Here's how the part is built. I have some questions about the finished solid (model axes, mm). A direction names the side the tool comes from. Give positions to 0.01 mm unless a question says otherwise; leave off trailing zeros. Write each loop counter-clockwise with the first axis right and the second up, starting at its lowest first coordinate (ties: lowest second). Pieces come first, ordered by that corner, then holes. Notation, with made-up numbers: (65, 41.5) -> (81, 41.5) arc R26 cw to (81, 80.5) -> close; hole circle Ø7 at (13.25, 32). An arc over 180 degrees is marked (long way). Use CSV: the item, a comma, the result in double quotes. Start each with the question number.
(1) For pin 1 Ø1 at (y, z) = (567, 48.5) entering from -X; pin 2 Ø21 at (x, y) = (339, 296) entering from +Z; pin 3 Ø21 at (x, y) = (336, 444) entering from -Z, each with a flat end and sliding along its axis, tell me the tip position at first contact or that it passes through.
(2) I need wall thicknesses on L1, parallel to X at y = 644.5, z = -14; L2, parallel to X at y = 35, z = 18.5; L3, parallel to Y at x = -117.5, z = -49.5. Which ranges of each line are inside material? Lowest first, please. Write a range as [from, to].
(3) Suppose I cut it at C-C on x = -142.5. List the corners of the cut face in (y, z) for me, plus the area to 3 significant figures.
(4) Which directions (+Z, -Z, +X, -X, +Y, -Y) give clear straight access to the entire face, cutting with the end or side of a thin tool? Please do faces 1 (the flat face through (364, 345, 28.85)), 2 (the flat face through (338, 345, 48.85)), 3 (the flat face through (338, 345, -31.15)).
(5) Suppose I cut it at B-B on z = 11. List the corners of the cut face in (x, y) for me, plus the area to 3 significant figures.
(6) Suppose I cut it at D-D on z = -52.5. List the corners of the cut face in (x, y) for me, plus the area to 3 significant figures.
(7) If we mould it in two halves opening along X, with no side actions, what happens to faces 4 (the flat face through (345, 698.9, 9)), 5 (the flat face through (-324.85, 345, 9)), 6 (the flat face through (350.95, 345, 39))? For each: pulls with the +X half, pulls with the -X half, needs draft (parallel to the pull), parting line crosses it, or undercut.
(8) Suppose I cut it at A-A on y = 478. List the corners of the cut face in (x, z) for me.
from build123d import *

# Parameters (mm, degrees)
F0_W     = 780.2
F0_H     = 122.3
F1_DEPTH = 26.1
F2_W     = 25
F2_H     = 40
F3_DEPTH = 698.9


with BuildPart() as f1:
    # F0 (on Front) → F1 (new body)
    with BuildSketch(Plane.XZ):
        Rectangle(F0_W, F0_H)
    extrude(amount=F1_DEPTH)

    # F2 (on face) → F3 (join)
    with BuildSketch(Plane(origin=(0, 0, 0), x_dir=(-1, 0, 0), z_dir=(0, 1, 0))):
        Polygon((-350.95, 48.85), (-350.95, 28.85), (-350.95, -11.15), (-350.95, -31.15), (-324.85, -31.15), (-324.85, 48.85), align=None)
        Polygon((350.95, 28.85), (350.95, 48.85), (324.85, 48.85), (324.85, -31.15), (350.95, -31.15), (350.95, -11.15), align=None)
        with Locations((363.45, 8.85)):
            Rectangle(F2_W, F2_H)
        with Locations((-363.45, 8.85)):
            Rectangle(F2_W, F2_H)
    extrude(amount=F3_DEPTH)


solid = f1.part
Geometry says:
1,pin 1,"x = -350.95"
1,pin 2,"z = 48.85"
1,pin 3,"z = -31.15"
2,L1,"[-350.95, -324.85], [324.85, 350.95]"
2,L2,"[-375.95, -324.85], [324.85, 375.95]"
2,L3,"[-26.1, 0]"
3,outline,"(-26.1, -61.15) -> (0, -61.15) -> (0, 61.15) -> (-26.1, 61.15) -> close"
3,area,"3,190 mm²"
4,face 1,"+Z, +X, +Y"
4,face 2,"+Z, +X, -X, +Y"
4,face 3,"-Z, +X, -X, +Y"
5,outline,"(-390.1, -26.1) -> (390.1, -26.1) -> (390.1, 0) -> (375.95, 0) -> (375.95, 698.9) -> (324.85, 698.9) -> (324.85, 0) -> (-324.85, 0) -> (-324.85, 698.9) -> (-375.95, 698.9) -> (-375.95, 0) -> (-390.1, 0) -> close"
5,area,"91,800 mm²"
6,outline,"(-390.1, -26.1) -> (390.1, -26.1) -> (390.1, 0) -> (-390.1, 0) -> close"
6,area,"20,400 mm²"
7,face 4,"needs draft"
7,face 5,"undercut"
7,face 6,"pulls with the +X half"
8,outline,"(-375.95, -11.15) -> (-350.95, -11.15) -> (-350.95, -31.15) -> (-324.85, -31.15) -> (-324.85, 48.85) -> (-350.95, 48.85) -> (-350.95, 28.85) -> (-375.95, 28.85) -> close; (324.85, -31.15) -> (350.95, -31.15) -> (350.95, -11.15) -> (375.95, -11.15) -> (375.95, 28.85) -> (350.95, 28.85) -> (350.95, 48.85) -> (324.85, 48.85) -> close"
